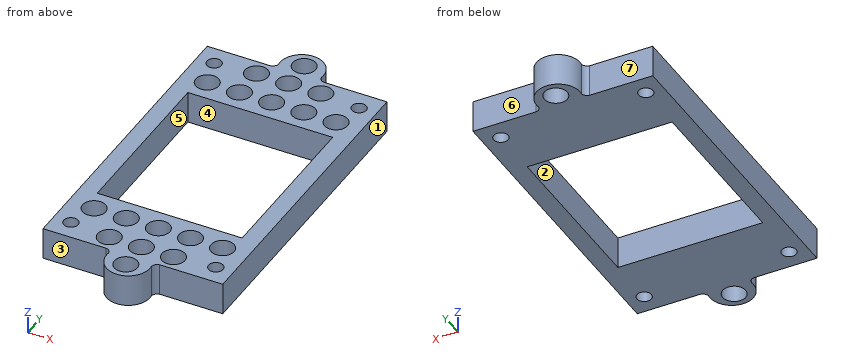
from build123d import *

# Parameters (mm, degrees)
SKETCH1_R           = 1.35
SKETCH1_R_2         = 2.15
SKETCH1_W           = 27
SKETCH1_H           = 32
BOSS_EXTRUDE1_DEPTH = 6
SKETCH2_R           = 2.15
CUT_EXTRUDE1_DEPTH  = 4.2


with BuildPart() as part:
    # Sketch1 → Boss-Extrude1 (new body)
    with BuildSketch(Plane.XY):
        with BuildLine():
            Line((-16.75, 29), (-5, 29))
            ThreePointArc((-5, 29), (-4.324155518, 29.324155518), (-4, 30))
            ThreePointArc((-4, 30), (0, 34.662885145), (4, 30))
            ThreePointArc((4, 30), (4.330169642, 29.330169642), (5, 29))
            Line((5, 29), (16.75, 29))
            Line((16.75, 29), (16.75, -29))
            Line((16.75, -29), (5, -29))
            ThreePointArc((5, -29), (4.330169642, -29.330169642), (4, -30))
            ThreePointArc((4, -30), (0, -34.662885145), (-4, -30))
            ThreePointArc((-4, -30), (-4.324155518, -29.324155518), (-5, -29))
            Line((-5, -29), (-16.75, -29))
            Line((-16.75, -29), (-16.75, 29))
        make_face()
        with Locations((-13.5, 25.3)):
            Circle(SKETCH1_R, mode=Mode.SUBTRACT)
        with Locations((13.5, -25.3)):
            Circle(SKETCH1_R, mode=Mode.SUBTRACT)
        with Locations((-13.5, -25.3)):
            Circle(SKETCH1_R, mode=Mode.SUBTRACT)
        with Locations((13.5, 25.3)):
            Circle(SKETCH1_R, mode=Mode.SUBTRACT)
        with Locations((0, 31.5)):
            Circle(SKETCH1_R_2, mode=Mode.SUBTRACT)
        with Locations(Location((0, -31.5, 0), (0, 0, 180))):
            Circle(SKETCH1_R_2, mode=Mode.SUBTRACT)
        Rectangle(SKETCH1_W, SKETCH1_H, mode=Mode.SUBTRACT)
    extrude(amount=BOSS_EXTRUDE1_DEPTH)

    # Sketch2 → Cut-Extrude1 (cut)
    with BuildSketch(Plane.XY.offset(6)):
        with Locations((-12, 20)):
            Circle(SKETCH2_R)
        with Locations((-6, 20)):
            Circle(SKETCH2_R)
        with Locations((0, 20)):
            Circle(SKETCH2_R)
        with Locations((6, 20)):
            Circle(SKETCH2_R)
        with Locations((12, 20)):
            Circle(SKETCH2_R)
        with Locations((-6, 26)):
            Circle(SKETCH2_R)
        with Locations((0, 26)):
            Circle(SKETCH2_R)
        with Locations((6, 26)):
            Circle(SKETCH2_R)
        with Locations((-11.967349369, -20)):
            Circle(SKETCH2_R)
        with Locations((-5.983674685, -20)):
            Circle(SKETCH2_R)
        with Locations((0, -20)):
            Circle(SKETCH2_R)
        with Locations((5.983674685, -20)):
            Circle(SKETCH2_R)
        with Locations((11.967349369, -20)):
            Circle(SKETCH2_R)
        with Locations((-5.983674685, -26)):
            Circle(SKETCH2_R)
        with Locations((0, -26)):
            Circle(SKETCH2_R)
        with Locations((5.983674685, -26)):
            Circle(SKETCH2_R)
    extrude(amount=-CUT_EXTRUDE1_DEPTH, mode=Mode.SUBTRACT)


solid = part.part
Work out the finished part from the listing and answer in its coordinate system (mm). Face numbers are marked on the shaded views. A direction names the side the tool comes from. Give positions to 0.01 mm unless a question says otherwise; leave off trailing zeros. Write each loop counter-clockwise with the first axis right and the second up, starting at its lowest first coordinate (ties: lowest second). Pieces come first, ordered by that corner, then holes. Notation, with made-up numbers: M 23.5,-7 L 37.5,-7 A32 ccw 37.5,31 Z; hole C 22,24.5 d5. An arc over 180 degrees is marked long. Answer as CSV lines item,"result".
Q1. A cutting plane is placed at D-D on x = -6. Write down the section's boundary in (y, z), plus the area to 3 significant figures.
A:
outline,"M -29,0 L -16,0 L -16,6 L -17.85,6 L -17.85,1.8 L -22.15,1.8 L -22.15,6 L -23.85,6 L -23.85,1.8 L -28.15,1.8 L -28.15,6 L -29,6 Z; M 16,0 L 29,0 L 29,6 L 28.15,6 L 28.15,1.8 L 23.85,1.8 L 23.85,6 L 22.15,6 L 22.15,1.8 L 17.85,1.8 L 17.85,6 L 16,6 Z"
area,"83.8 mm²"
Q2. A cutting plane is placed at B-B on y = -7.5. Write down the section's boundary in (x, z).
A:
outline,"M -16.75,0 L -13.5,0 L -13.5,6 L -16.75,6 Z; M 13.5,0 L 16.75,0 L 16.75,6 L 13.5,6 Z"
Q3. Find the intervals of material crossed by probe 1 along X at (y, z) = (-3, 3.95); probe 2 along Y at (x, z) = (7.5, 0.35); probe 3 along Y at (x, z) = (11, 5), in increasing order. Write a range as [from, to].
A:
probe 1,"x = [-16.75, -13.5], [13.5, 16.75]"
probe 2,"y = [-29, -16], [16, 29]"
probe 3,"y = [-29, -21.92], [-18.08, -16], [16, 18.1], [21.9, 29]"
Q4. A cutting plane is placed at C-C on y = -25.3. Write down the section's boundary in (x, z), plus the area to 3 significant figures.
A:
outline,"M -16.75,0 L -14.85,0 L -14.85,6 L -16.75,6 Z; M -12.15,0 L 12.15,0 L 12.15,6 L 8.02,6 L 8.02,1.8 L 3.95,1.8 L 3.95,6 L 2.03,6 L 2.03,1.8 L -2.03,1.8 L -2.03,6 L -3.95,6 L -3.95,1.8 L -8.02,1.8 L -8.02,6 L -12.15,6 Z; M 14.85,0 L 16.75,0 L 16.75,6 L 14.85,6 Z"
area,"117 mm²"
Q5. A tool of negligible diameter and unlimited length cuts with its end or side. For the marked faces 5, 6 and 7, from which of +Z, -Z, +X, -X, +Y, -Y can it reach the whole face along a straight path? Write none if from no direction.
A:
face 5,"+Z, -Z"
face 6,"+Z, -Z, +X, +Y"
face 7,"+Z, -Z, -X, +Y"
Q6. A cutting plane is placed at A-A on x = 0. Count the separate pieces of the cut face and the enclosed holes in it, plus the area to 3 significant figures.
A:
separate pieces,"4"
enclosed holes,"0"
area,"100 mm²"
Q7. The mould has two halves that part along Y. Classify the marked faces 1, 2, 3 and 4: +Y half, -Y half, draft (parallel to the pull), parting line (faces both ways), or undercut.
A:
face 1,"draft"
face 2,"undercut"
face 3,"-Y half"
face 4,"undercut"
Q8. Given P1, Ø3.5, axis at x = -6, y = 26, coming from the +Z side; P2, Ø3, axis at x = -9.5, z = 2.5, coming from the +Y side, each flat-ended and moving along its own axis, determine where each tip first touches the part or whether it passes through.
A:
P1,"stops at z = 1.8"
P2,"stops at y = 29"
